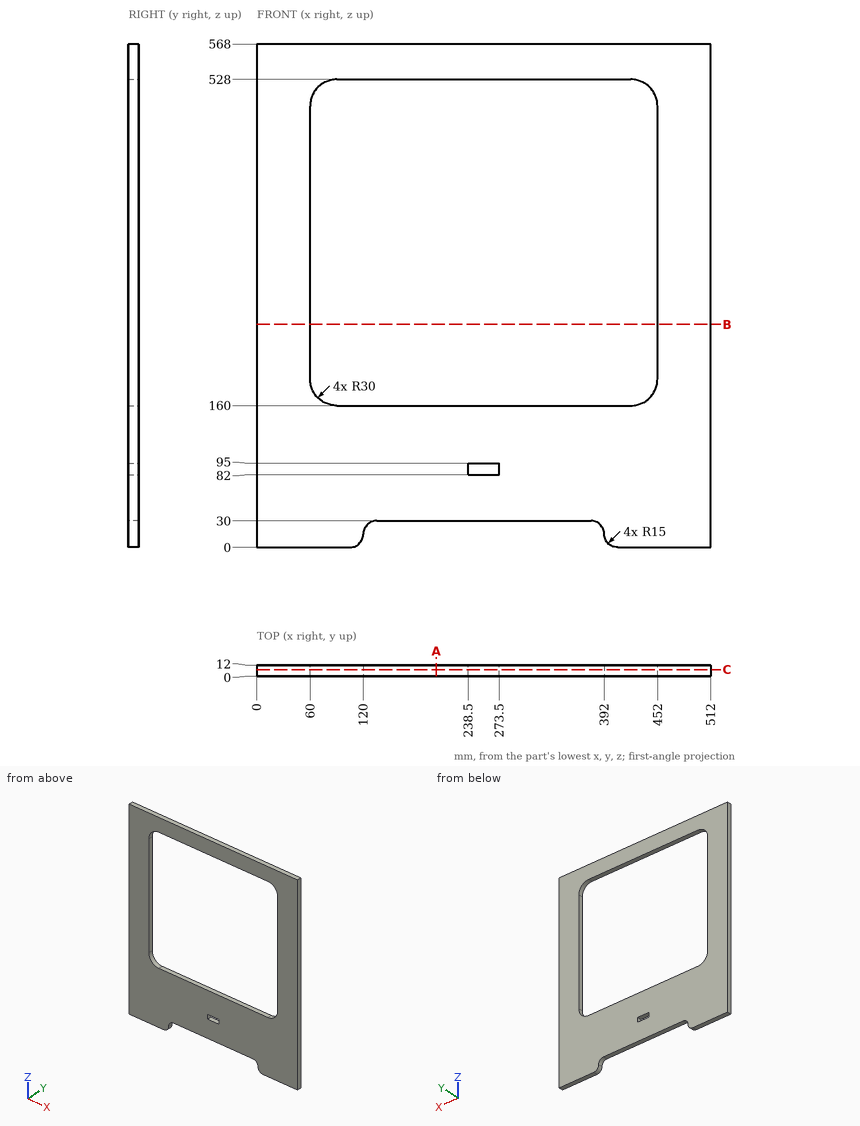
Source: three-view drawing plus pictorial views. Frame: mm from the lowest corner of the part. Round coordinates to 2 decimals unless told otherwise and drop trailing zeros. Order: outer loops, then holes, each group sorted by start corner. A loop starts at its lowest first (then second) coordinate and runs counter-clockwise, first axis right, second up. Notation, with made-up numbers: M 47,39 L 70,39 A27 cw 70,77 Z; hole C 60.5,-2 d10. An arc over 180 degrees is marked long. One line per item, written item: value.
(1) Cut plane C-C (y = 7.25). Give the number of separate pieces and of enclosed holes in the cut face, and give its area (3 significant figures).
Result sheet:
separate pieces: 1
enclosed holes: 2
area: 139,000 mm2
(2) Cut plane B-B (z = 251.5). Return the cut outline in (x, y), and give its area (3 significant figures).
Result sheet:
outline: M 0,0 L 60,0 L 60,12 L 0,12 Z; M 452,0 L 512,0 L 512,12 L 452,12 Z
area: 1,440 mm2
(3) Pin query (flat end, axial travel): P1, Ø3, axis at x = 119.5, y = 8, coming from the -Z side; P2, Ø3, axis at y = 7, z = 137, coming from the -X side; P3, Ø3.5, axis at x = 240.5, y = 7.5, coming from the -Z side. Return the tip coordinate at first contact, or that it passes through.
Result sheet:
P1: z = 7.52
P2: x = 0
P3: z = 30
(4) Cut plane A-A (x = 202.5). Return the cut outline in (y, z), and give its area (3 significant figures).
Result sheet:
outline: M 0,30 L 12,30 L 12,160 L 0,160 Z; M 0,528 L 12,528 L 12,568 L 0,568 Z
area: 2,040 mm2
(5) Line query: probe 1 along Z at (x, y) = (240, 2); probe 2 along Z at (x, y) = (101, 3.5); probe 3 along Z at (x, y) = (351.5, 2.75). Output: solid intervals per line, ascending. Write a range as [from, to].
Result sheet:
probe 1: [30, 82], [95, 160], [528, 568]
probe 2: [0, 160], [528, 568]
probe 3: [30, 160], [528, 568]
